Input: part model. Units: mm. Frame: model coordinates. Coordinates: 2 decimals unless noted, no trailing zeros. Order: outer loops, then holes, each group sorted by start corner. A loop starts at its lowest first (then second) coordinate and runs counter-clockwise, first axis right, second up.
from build123d import *

# Parameters (mm, degrees)
F0_W     = 140
F0_H     = 59
F1_DEPTH = 3.3
F2_R     = 1.5
F3_DEPTH = 25
F4_SIZE  = 2


with BuildPart() as f1:
    # F0 (on Front) → F1 (new body)
    with BuildSketch(Plane.XZ):
        Rectangle(F0_W, F0_H)
        Polygon((85, -29.5), (70, 29.5), (70, -29.5), align=None)
    extrude(amount=F1_DEPTH)

    # F2 (on face) → F3 (cut)
    with BuildSketch(Plane.XZ.offset(3.3)):
        with Locations((-55, 14.5)):
            Circle(F2_R)
        with Locations((63, 14.5)):
            Circle(F2_R)
        with Locations((63, -9.5)):
            Circle(F2_R)
        with Locations((-55, -9.5)):
            Circle(F2_R)
    extrude(amount=-F3_DEPTH, mode=Mode.SUBTRACT)

    # F4
    f4_edges = [f1.edges().sort_by_distance(p)[0] for p in [
        (-56.5, 0, -9.5),
        (-56.5, 0, 14.5),
        (61.5, 0, -9.5),
        (61.5, 0, 14.5),
    ]]
    chamfer(f4_edges, length=F4_SIZE)


solid = f1.part
Item 1: Cut plane C-C on z = 14.5. Return loops of the section in (x, y), then the cut area to 3 significant figures.
Response values:
outline: (-70, -3.3) - (-56.5, -3.3) - (-56.5, -2) - (-58.5, 0) - (-70, 0) - close; (-53.5, -3.3) - (61.5, -3.3) - (61.5, -2) - (59.5, 0) - (-51.5, 0) - (-53.5, -2) - close; (64.5, -3.3) - (73.81, -3.3) - (73.81, 0) - (66.5, 0) - (64.5, -2) - close
area: 447 mm2
Item 2: Draft query along Z for faces 1 (the face through (-1, -2, 29.5)), 2 (the face through (6, 0, 0)), 3 (the face through (-53.614, -2.659, -10.075)), 4 (the face through (6, -2, -29.5)). Return one class per face: pulls with the +Z half, pulls with the -Z half, needs draft (parallel to the pull), parting line crosses it, or undercut.
Response values:
face 1: pulls with the +Z half
face 2: needs draft
face 3: undercut
face 4: pulls with the -Z half
Item 3: Cut plane D-D on z = 21. Return loops of the section in (x, y).
Response values:
outline: (-70, -3.3) - (72.16, -3.3) - (72.16, 0) - (-70, 0) - close
Item 4: Pin query (flat end, axial travel): pin 1 Ø5 at (x, z) = (63, 14.5) entering from -Y; pin 2 Ø4 at (x, z) = (63, -9.5) entering from +Y; pin 3 Ø2.5 at (x, z) = (-55, -9.5) entering from +Y. Return the tip coordinate at first contact, or that it passes through.
Response values:
pin 1: stops at y = -3.3
pin 2: stops at y = -1.5
pin 3: passes through
Item 5: Cut plane B-B on y = -1.05. Return loops of the section in (x, z), then the cut area to 3 significant figures.
Response values:
outline: (-70, -29.5) - (85, -29.5) - (70, 29.5) - (-70, 29.5) - close; hole circle Ø4.9 at (-55, -9.5); hole circle Ø4.9 at (-55, 14.5); hole circle Ø4.9 at (63, -9.5); hole circle Ø4.9 at (63, 14.5)
area: 8,630 mm2
Item 6: Cut plane A-A on x = -55. Return loops of the section in (y, z), then the cut area to 3 significant figures.
Response values:
outline: (-3.3, -29.5) - (0, -29.5) - (0, -13) - (-2, -11) - (-3.3, -11) - close; (-3.3, -8) - (-2, -8) - (0, -6) - (0, 11) - (-2, 13) - (-3.3, 13) - close; (-3.3, 16) - (-2, 16) - (0, 18) - (0, 29.5) - (-3.3, 29.5) - close
area: 167 mm2
Item 7: Ray query, probe 1 along Z at (x, y) = (-55, -2.25); probe 2 along X at (y, z) = (-0.25, 15); probe 3 along X at (y, z) = (-3.1, -15). Return the intervals inside material, ascending.
Response values:
probe 1: z = -29.5 to -11, -8 to 13, 16 to 29.5
probe 2: x = -70 to -58.21, -51.79 to 59.79, 66.21 to 73.69
probe 3: x = -70 to 81.31
